Verification items for the finished model (mm, model axes). Give positions to 0.01 mm unless a question says otherwise; leave off trailing zeros. Loops run counter-clockwise (first coordinate to the right, second up) from the corner with the lowest first, then second, coordinate; pieces in that order, holes last. Notation, with made-up numbers: M 39.25,75 L 50.25,75 A23 ccw 50.25,101 Z; hole C 43,65 d8. An arc over 180 degrees is marked long. Answer in a Markdown table with one row per item.
Autodesk Inventor part; units mm, degrees
ref_plane "YZ Plane" through (0, 0, 0) normal (1, 0, 0) x (0, 1, 0)
ref_plane "XZ Plane" through (0, 0, 0) normal (0, 1, 0) x (-1, 0, 0)
ref_plane "XY Plane" through (0, 0, 0) normal (0, 0, 1) x (1, 0, 0)
sketch "Sketch1" plane through (0, 0, 0) normal (0, 0, 1) x (1, 0, 0)
  line L0 (0, 0) -> (203.2, 0)
  line L1 (203.2, 0) -> (203.2, 431.8)
  line L2 (203.2, 431.8) -> (170.815, 431.8)
  line L3 (0, 431.8) -> (0, 0)
  circle A0 centre (177.8, 406.4) radius 3.3782
  circle A1 centre (177.8, 215.9) radius 3.3782
  circle A2 centre (177.8, 25.4) radius 3.3782
  line L4 (203.2, 215.9) -> (0, 215.9) construction
  line L5 (94.615, 431.8) -> (145.415, 393.7)
  line L6 (145.415, 393.7) -> (170.815, 393.7)
  line L7 (170.815, 393.7) -> (170.815, 431.8)
  line L8 (94.615, 431.8) -> (0, 431.8)
  line L9 (170.815, 431.8) -> (94.615, 431.8)
  circle A3 centre (139.7, 304.8) radius 2.3495
  line L10 (139.7, 304.8) -> (139.7, 246.634) construction
  circle A4 centre (139.7, 246.634) radius 2.3495
  circle A5 centre (45.6, 310.6) radius 2.54
  circle A6 centre (38.1, 292.1) radius 2.54
  line L11 (45.6, 310.6) -> (38.1, 310.6) construction
  line L12 (38.1, 310.6) -> (38.1, 292.1) construction
  line L13 (38.1, 292.1) -> (45.6, 292.1) construction
  line L14 (45.6, 292.1) -> (45.6, 310.6) construction
  circle A7 centre (38.1, 12.7) radius 2.3495
  line L15 (71.1544, 389.1684) -> (109.2544, 389.1684) construction
  line L16 (109.2544, 389.1684) -> (109.2544, 370.1184) construction
  line L17 (109.2544, 370.1184) -> (71.1544, 370.1184) construction
  line L18 (71.1544, 370.1184) -> (71.1544, 389.1684) construction
  line L19 (95.25, 165.1) -> (152.4, 165.1) construction
  line L20 (152.4, 165.1) -> (152.4, 50.8) construction
  line L21 (152.4, 50.8) -> (95.25, 50.8) construction
  line L22 (95.25, 50.8) -> (95.25, 165.1) construction
  circle A8 centre (95.25, 165.1) radius 3.175
  circle A9 centre (152.4, 165.1) radius 3.175
  circle A10 centre (152.4, 50.8) radius 3.175
  circle A11 centre (95.25, 50.8) radius 3.175
  line L23 (30.6, 229.55) -> (30.6, 259.55)
  arc A12 (30.6, 229.55) -> (34.6, 225.55) centre (34.6, 229.55) ccw
  line L24 (52.6, 225.55) -> (34.6, 225.55)
  line L25 (52.6, 225.55) -> (52.6, 263.55)
  line L26 (34.6, 263.55) -> (52.6, 263.55)
  arc A13 (34.6, 263.55) -> (30.6, 259.55) centre (34.6, 259.55) ccw
  arc A14 (49.81, 256.2) -> (44.31, 256.2) centre (47.06, 256.2) ccw
  line L27 (49.81, 256.2) -> (49.81, 248.7)
  arc A15 (44.31, 248.7) -> (49.81, 248.7) centre (47.06, 248.7) ccw
  line L28 (44.31, 248.7) -> (44.31, 256.2)
  arc A16 (41.85, 240.2) -> (36.35, 240.2) centre (39.1, 240.2) ccw
  line L29 (41.85, 240.2) -> (41.85, 232.7)
  arc A17 (36.35, 232.7) -> (41.85, 232.7) centre (39.1, 232.7) ccw
  line L30 (36.35, 232.7) -> (36.35, 240.2)
  circle A18 centre (30.4488, 139.597) radius 2.3812
  circle A19 centre (64.8012, 139.597) radius 2.3812
  circle A20 centre (30.4488, 106.323) radius 2.3812
  circle A21 centre (64.8012, 106.323) radius 2.3812
  dimension "d0" = 6.7564
  dimension "d3" = 190.5
  dimension "d8" = 25.4
  dimension "d9" = 431.8
  dimension "d10" = 203.2
  dimension "d14" = 38.1
  dimension "d15" = 76.2
  dimension "d16" = 25.4
  dimension "d17" = 4.699
  dimension "d18" = 58.166
  dimension "d19" = 63.5
  dimension "d20" = 127
  dimension "d26" = 5.08
  dimension "d27" = 18.5
  dimension "d28" = 7.5
  dimension "d29" = 38.1
  dimension "d30" = 76.2
  dimension "d31" = 4.699
  dimension "d32" = 38.1
  dimension "d33" = 12.7
  dimension "d34" = 32.385
  dimension "d35" = 19.05
  dimension "d36" = 38.1
  dimension "d37" = 57.15
  dimension "d38" = 6.35
  dimension "d39" = 114.3
  dimension "d40" = 50.8
  dimension "d41" = 50.8
extrude "Extrusion1" add sketch "Sketch1" along normal blind 3.175 contours L3 L8 L5 L6 L7 L2 L1 L0 | L23 A13 L26 L25 L24 A12
properties part number "Electrical Board 2" material "Polycarbonate, Clear"
Item 1: Sectioned sample at A-A (z = 2). State how many separate pieces and enclosed holes the cut face has, and give its area (3 significant figures).
Reported:
| item | result |
|---|---|
| separate pieces | 1 |
| enclosed holes | 18 |
| area | 85,300 mm^2 |
Item 2: Scan lines: L1, parallel to X at y = 165.1, z = 1.5 (3 decimals); L2, parallel to X at y = 139.5, z = 3.05; L3, parallel to Y at x = 152.4, z = 0.7 (3 decimals). Record each from-to range of solid material in increasing order. Write a range as [from, to].
Reported:
| item | result |
|---|---|
| L1 | x = [0, 92.075], [98.425, 149.225], [155.575, 203.2] |
| L2 | x = [0, 28.07], [32.83, 62.42], [67.18, 203.2] |
| L3 | y = [0, 47.625], [53.975, 161.925], [168.275, 393.7] |
Item 3: Release check for a two-part mould opening along X. For faces 1 (the flat face through (119.659, 413.017, 1.565)), 2 (the flat face through (100, 219, 3.175)) record: released by +X, released by -X, zero draft, split by the parting line, or undercut.
Reported:
| item | result |
|---|---|
| face 1 | undercut |
| face 2 | zero draft |
Item 4: Sectioned sample at B-B (x = 111). Record the cut outline in (y, z) (3 decimals), and give its area (3 significant figures).
Reported:
| item | result |
|---|---|
| outline | M 0,0 L 419.511,0 L 419.511,3.175 L 0,3.175 Z |
| area | 1,330 mm^2 |
Item 5: Go/stop test with a flat-tipped pin: pin 1 (1 mm diameter, centred on x = 160.5, z = 2, fed in from +Y). Record where the tip stops, or that it passes through.
Reported:
| item | result |
|---|---|
| pin 1 | stops at y = 393.7 |
